```python
from build123d import *

# Parameters (mm, degrees)
SKETCH_1_W          = 300
SKETCH_1_H          = 10
SKETCH_1_R          = 1.558433933
EXTRUDE_4_DEPTH     = 10
SKETCH_5_R          = 1.5
CUT_EXTRUDE_1_DEPTH = 10
SKETCH_9_W          = 8
SKETCH_9_H          = 8
CUT_EXTRUDE_4_DEPTH = 300


with BuildPart() as part:
    # 草图1 → 凸台-拉伸4 (new body)
    with BuildSketch(Plane(origin=(0, 0, 0), x_dir=(0, 0, -1), z_dir=(1, 0, 0))):
        with Locations((95.027173063, 0.135119806)):
            Rectangle(SKETCH_1_W, SKETCH_1_H)
        with Locations((-39.972826937, 0.135119806)):
            Circle(SKETCH_1_R, mode=Mode.SUBTRACT)
        with Locations((-29.972826937, 0.135119806)):
            Circle(SKETCH_1_R, mode=Mode.SUBTRACT)
        with Locations((-19.972826937, 0.135119806)):
            Circle(SKETCH_1_R, mode=Mode.SUBTRACT)
        with Locations((210.027173063, 0.135119806)):
            Circle(SKETCH_1_R, mode=Mode.SUBTRACT)
        with Locations((220.027173063, 0.135119806)):
            Circle(SKETCH_1_R, mode=Mode.SUBTRACT)
        with Locations((230.027173063, 0.135119806)):
            Circle(SKETCH_1_R, mode=Mode.SUBTRACT)
    extrude(amount=EXTRUDE_4_DEPTH)

    # 草图5 → 切除-拉伸1 (cut)
    with BuildSketch(Plane(origin=(10, 0, 0), x_dir=(0, 0, -1), z_dir=(1, 0, 0))):
        with Locations((95.027173063, 0.135119806)):
            Circle(SKETCH_5_R)
    extrude(amount=-CUT_EXTRUDE_1_DEPTH, mode=Mode.SUBTRACT)

    # 草图9 → 切除-拉伸4 (cut)
    with BuildSketch(Plane.XY.offset(54.972826937)):
        with Locations((5, 0.135119806)):
            Rectangle(SKETCH_9_W, SKETCH_9_H)
    extrude(amount=-CUT_EXTRUDE_4_DEPTH, mode=Mode.SUBTRACT)


solid = part.part
```
The model under review builds one solid part; all positions refer to its coordinate system, in mm. A direction names the side the tool comes from. Round coordinates to 2 decimals unless told otherwise and drop trailing zeros. Order: outer loops, then holes, each group sorted by start corner. A loop starts at its lowest first (then second) coordinate and runs counter-clockwise, first axis right, second up. Notation, with made-up numbers: M 68.25,59 L 76.25,59 A22 cw 76.25,70 Z; hole C 3.5,-32.5 d3. An arc over 180 degrees is marked long. Use a Markdown table: item, result.
1) Consider section A-A (z = -61.5). Write out the cut boundary in (x, y), then the cut area to 3 significant figures.
Report:
| item | result |
|---|---|
| outline | M 0,-4.86 L 10,-4.86 L 10,5.14 L 0,5.14 Z; hole M 1,-3.86 L 9,-3.86 L 9,4.14 L 1,4.14 Z |
| area | 36.0 mm^2 |
2) Draft analysis for pull direction X (two halves, no side actions). For faces 1 (the face through (0, 0, -93)), 2 (the face through (9.4, 0.1, -245.027)), 3 (the face through (5, -3.865, -93)), state which applies: released by +X, released by -X, zero draft, split by the parting line, or undercut.
Report:
| item | result |
|---|---|
| face 1 | released by -X |
| face 2 | zero draft |
| face 3 | undercut |
3) Consider section B-B (x = 7.5). Write out the cut boundary in (y, z), then the cut area to 3 significant figures.
Report:
| item | result |
|---|---|
| outline | M -4.86,-245.03 L -3.86,-245.03 L -3.86,54.97 L -4.86,54.97 Z; M 4.14,-245.03 L 5.14,-245.03 L 5.14,54.97 L 4.14,54.97 Z |
| area | 600 mm^2 |
4) Tool access review of faces 4 (the face through (5, -4.865, -93)), 5 (the face through (5, 4.135, -93)): name each direction out of +Z, -Z, +X, -X, +Y, -Y from which nothing blocks a thin tool from reaching the whole face with its end or side.
Report:
| item | result |
|---|---|
| face 4 | +Z, -Z, +X, -X, -Y |
| face 5 | +Z, -Z |
5) Wall thickness on line 1 along Y through (x, z) = (7.75, -81); line 2 along Y through (x, z) = (0.75, -95); line 3 along X through (y, z) = (0.5, 25): over which ranges is each line inside the solid? List them lowest first. Write a range as [from, to].
Report:
| item | result |
|---|---|
| line 1 | [-4.86, -3.86], [4.14, 5.14] |
| line 2 | [-4.86, -1.36], [1.63, 5.14] |
| line 3 | [0, 1], [9, 10] |
